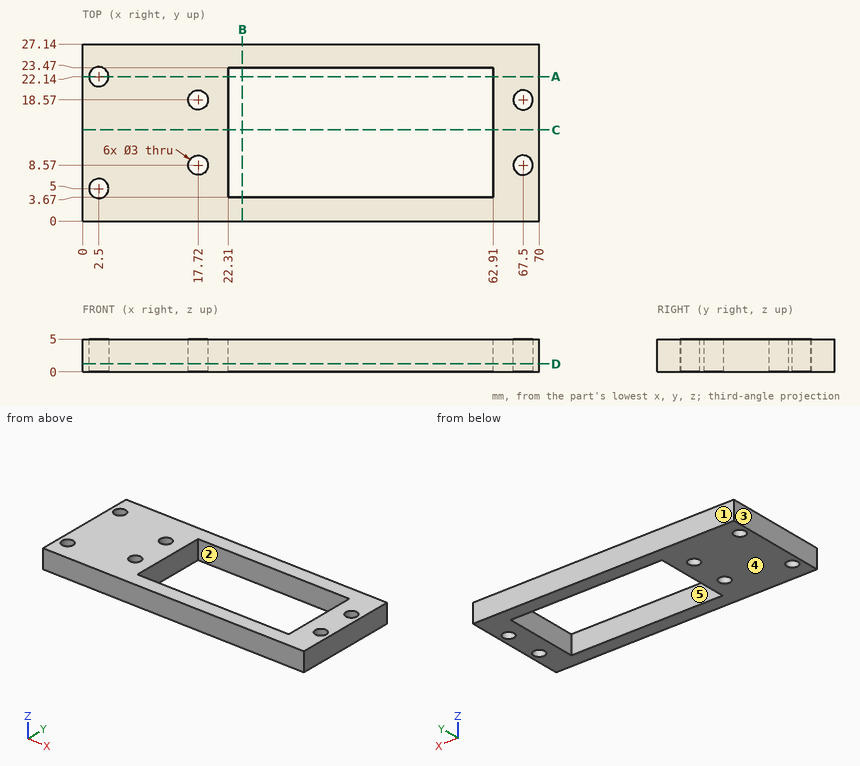
The drawing under review shows one solid part. Ordinate dimensions are in mm from its lowest x, y, z. A direction names the side the tool comes from. Coordinates: 2 decimals unless noted, no trailing zeros. Write each loop counter-clockwise with the first axis right and the second up, starting at its lowest first coordinate (ties: lowest second). Pieces come first, ordered by that corner, then holes. Notation, with made-up numbers: (21, 21) -> (60, 21) arc R7 ccw to (60, 28) -> close; hole circle Ø1 at (-13.5, 35). An arc over 180 degrees is marked (long way). Write each question's results on one line, items separated by ' | '. Start each with the question number.
1) Insertion check: pin 1 (1.5 mm diameter, centred on x = 23.5, y = 23, fed in from +Z); pin 2 (1.8 mm diameter, centred on x = 67.5, y = 8.57, fed in from -Z). Each pin has a flat end and moves straight along its axis. Give the tip position at first contact, or say it passes through.
2) Consider section D-D (z = 1.2). Write out the cut boundary in (x, y).
3) Consider section B-B (x = 24.5). Write out the cut boundary in (y, z).
4) Consider section A-A (y = 22.14). Write out the cut boundary in (x, z), plus the area to 3 significant figures.
5) Wall thickness on L1, parallel to Y at x = 2.5, z = 3.7; L2, parallel to X at y = 8.5, z = 4.85; L3, parallel to X at y = 22, z = 4.2: over which ranges is each line inside the solid? List them lowest first. Write a range as [from, to].
6) For the marked faces 4 and 5, list the 3-axis set-ups (+Z, -Z, +X, -X, +Y, -Y) from which the entire face can be reached by the end or side of a thin tool; tool diameter is ignored.
7) The part is to be moulded in two halves that separate along X. For the marked faces 1, 2 and 3, say which applies: +X half, -X half, draft (parallel to the pull), parting line (faces both ways), or undercut.
8) Consider section C-C (y = 14). Write out the cut boundary in (x, z), plus the area to 3 significant figures.
Geometry says:
1) pin 1: z = 5 | pin 2: through
2) outline: (0, 0) -> (70, 0) -> (70, 27.14) -> (0, 27.14) -> close; hole circle Ø3 at (2.5, 5); hole circle Ø3 at (2.5, 22.14); hole circle Ø3 at (17.72, 8.57); hole circle Ø3 at (17.72, 18.57); hole (22.31, 3.67) -> (62.91, 3.67) -> (62.91, 23.47) -> (22.31, 23.47) -> close; hole circle Ø3 at (67.5, 8.57); hole circle Ø3 at (67.5, 18.57)
3) outline: (0, 0) -> (3.67, 0) -> (3.67, 5) -> (0, 5) -> close; (23.47, 0) -> (27.14, 0) -> (27.14, 5) -> (23.47, 5) -> close
4) outline: (0, 0) -> (1, 0) -> (1, 5) -> (0, 5) -> close; (4, 0) -> (22.31, 0) -> (22.31, 5) -> (4, 5) -> close; (62.91, 0) -> (70, 0) -> (70, 5) -> (62.91, 5) -> close | area: 132 mm^2
5) L1: [0, 3.5], [6.5, 20.64], [23.64, 27.14] | L2: [0, 16.22], [19.22, 22.31], [62.91, 66], [69, 70] | L3: [0, 1.01], [3.99, 22.31], [62.91, 70]
6) face 4: -Z, +X, -X, +Y, -Y | face 5: +Z, -Z
7) face 1: draft | face 2: undercut | face 3: -X half
8) outline: (0, 0) -> (22.31, 0) -> (22.31, 5) -> (0, 5) -> close; (62.91, 0) -> (70, 0) -> (70, 5) -> (62.91, 5) -> close | area: 147 mm^2
